```python
from build123d import *

# Parameters (mm, degrees)
F0_W     = 42.3
F0_H     = 42.3
F0_R     = 2.5
F0_R_2   = 11
F1_DEPTH = 48
F2_DEPTH = 5
F3_DEPTH = 2
F4_DEPTH = 24


with BuildPart() as f1:
    # F0 (on Front) → F1 (new body)
    with BuildSketch(Plane.XZ):
        Rectangle(F0_W, F0_H)
        with Locations((-15.5, -15.5)):
            Circle(F0_R, mode=Mode.SUBTRACT)
        with Locations((15.5, -15.5)):
            Circle(F0_R, mode=Mode.SUBTRACT)
        with Locations((-15.5, 15.5)):
            Circle(F0_R, mode=Mode.SUBTRACT)
        Circle(F0_R_2, mode=Mode.SUBTRACT)
        with Locations((15.5, 15.5)):
            Circle(F0_R, mode=Mode.SUBTRACT)
        Circle(F0_R_2)
        Circle(F0_R, mode=Mode.SUBTRACT)
        with Locations((-15.5, 15.5)):
            Circle(F0_R)
        Circle(F0_R)
        with Locations((15.5, 15.5)):
            Circle(F0_R)
        with Locations((-15.5, -15.5)):
            Circle(F0_R)
        with Locations((15.5, -15.5)):
            Circle(F0_R)
    extrude(amount=-F1_DEPTH)

    # F0 (on Front) → F2 (cut)
    with BuildSketch(Plane.XZ):
        with Locations((-15.5, 15.5)):
            Circle(F0_R)
        with Locations((15.5, 15.5)):
            Circle(F0_R)
        with Locations((15.5, -15.5)):
            Circle(F0_R)
        with Locations((-15.5, -15.5)):
            Circle(F0_R)
    extrude(amount=-F2_DEPTH, mode=Mode.SUBTRACT)

    # F0 (on Front) → F3 (join)
    with BuildSketch(Plane.XZ):
        Circle(F0_R_2)
        Circle(F0_R, mode=Mode.SUBTRACT)
    extrude(amount=F3_DEPTH)

    # F0 (on Front) → F4 (join)
    with BuildSketch(Plane.XZ):
        Circle(F0_R)
    extrude(amount=F4_DEPTH)


solid = f1.part
```
Could you check a few things on this model? Use its own coordinates, in mm. A direction names the side the tool comes from. Give positions to 0.01 mm unless a question says otherwise; leave off trailing zeros. Loops run counter-clockwise (first coordinate to the right, second up) from the corner with the lowest first, then second, coordinate; pieces in that order, holes last. Notation, with made-up numbers: (33.25, -38.5) -> (66.25, -38.5) arc R23 ccw to (66.25, -13.5) -> close; hole circle Ø6 at (75, -5). An arc over 180 degrees is marked (long way). Put each result on its own line as item: value.
(1) Imagine slicing it at B-B on x = -15.5. Write out the boundary of the cut face in (y, z), plus the area to 3 significant figures.
Computed:
outline: (0, -21.15) -> (48, -21.15) -> (48, 21.15) -> (0, 21.15) -> (0, 18) -> (5, 18) -> (5, 13) -> (0, 13) -> (0, -13) -> (5, -13) -> (5, -18) -> (0, -18) -> close
area: 1,980 mm^2
(2) For faces 4 (the face through (0, -24, 0)), 5 (the face through (-17.5, 2.5, -17)), which set-ups out of +Z, -Z, +X, -X, +Y, -Y let a thin tool reach every point of the face, with its end or its side?
Computed:
face 4: +Z, -Z, +X, -X, -Y
face 5: -Y
(3) Please list where these lines run through material, in increasing order: probe 1 along Z at (x, y) = (-15.5, 1.7); probe 2 along Z at (x, y) = (15, 1). Write a range as [from, to].
Computed:
probe 1: [-21.15, -18], [-13, 13], [18, 21.15]
probe 2: [-21.15, -17.95], [-13.05, 13.05], [17.95, 21.15]
(4) Imagine slicing it at C-C on y = -7.5. Write out the boundary of the cut face in (x, z), plus the area to 3 significant figures.
Computed:
outline: circle Ø5 at (0, 0)
area: 19.6 mm^2
(5) Imagine slicing it at D-D on z = 9. Write out the boundary of the cut face in (x, y), plus the area to 3 significant figures.
Computed:
outline: (-21.15, 0) -> (-6.32, 0) -> (-6.32, -2) -> (6.32, -2) -> (6.32, 0) -> (21.15, 0) -> (21.15, 48) -> (-21.15, 48) -> close
area: 2,060 mm^2
(6) I'm going to push flat-ended pins straight in: pin 1 Ø12 at (x, z) = (-0.5, 9) entering from -Y; pin 2 Ø1.5 at (x, z) = (16.5, -14.5) entering from -Y; pin 3 Ø1 at (x, z) = (-4, -12) entering from -Y; pin 4 Ø10 at (y, z) = (-10, 16.5) entering from -X. Where does each tip first touch, or does it pass through?
Computed:
pin 1: y = -2
pin 2: y = 5
pin 3: y = 0
pin 4: through
(7) Imagine slicing it at A-A on z = 17. Write out the boundary of the cut face in (x, y), plus the area to 3 significant figures.
Computed:
outline: (-21.15, 0) -> (-17.5, 0) -> (-17.5, 5) -> (-13.5, 5) -> (-13.5, 0) -> (13.5, 0) -> (13.5, 5) -> (17.5, 5) -> (17.5, 0) -> (21.15, 0) -> (21.15, 48) -> (-21.15, 48) -> close
area: 1,990 mm^2
(8) Thinking about a two-plate mould opening in X: for faces 1 (the face through (0, 24, -21.15)), 2 (the face through (21.15, 24, 0)), 3 (the face through (15, 5, 16)), which applies, pulls with the +X half, pulls with the -X half, needs draft (parallel to the pull), parting line crosses it, or undercut?
Computed:
face 1: needs draft
face 2: pulls with the +X half
face 3: undercut
